For this review, take the finished solid that the model builds, in its own axes (mm). A direction names the side the tool comes from. Round coordinates to 2 decimals unless told otherwise and drop trailing zeros. Loops run counter-clockwise (first coordinate to the right, second up) from the corner with the lowest first, then second, coordinate; pieces in that order, holes last. Notation, with made-up numbers: M 69,71 L 106,71 A13 cw 106,79 Z; hole C -1,79.25 d1. An arc over 180 degrees is marked long. One line per question, with ' | ' between items. Start each with the question number.
1) For faces 5 (the face through (-1, -250, 42)), 6 (the face through (6, -30, -20)), 7 (the face through (-14, -140, 9)), list the 3-axis set-ups (+Z, -Z, +X, -X, +Y, -Y) from which the entire face can be reached by the end or side of a thin tool; tool diameter is ignored.
2) For pin 1 Ø5 at (x, y) = (-11.5, -99) entering from -Z; pin 2 Ø20 at (x, z) = (-17.5, 7.5) entering from -Y; pin 3 Ø2 at (x, y) = (-46.5, -216.5) entering from -Z, all flat-tipped, find the tip position at first contact; note any pin that passes through.
3) We need section C-C (y = -127). Give the boundary of the cut face in (x, z).
4) For probe 1 along Z at (x, y) = (2, -223.5); probe 2 along Z at (x, y) = (0, -29); probe 3 along Y at (x, z) = (34.5, -45.5), list the stretches that pass through material, from the lowest coordinate up. Write a range as from..to.
5) We need section A-A (x = 0). Give the boundary of the cut face in (y, z).
6) We need section B-B (z = 0). Give the boundary of the cut face in (x, y).
7) Mouldability with a two-part tool opening along Z and no side actions: class faces 1 (the face through (-1, -201, -30)), 2 (the face through (-4.336, -14.79, -19.524)), 3 (the face through (-14.985, -70.98, 0.66)), 4 (the face through (3, 0, 15)) as pulls with the +Z half, pulls with the -Z half, needs draft (parallel to the pull), parting line crosses it, or undercut.
8) We need section D-D (z = -23.5). Give the boundary of the cut face in (x, y).
```python
from build123d import *

# Parameters (mm, degrees)
F0_R     = 20
F1_DEPTH = 30
F2_R     = 30
F3_DEPTH = 40
F4_R     = 60
F5_DEPTH = 180
F6_R     = 15
F7_DEPTH = 250
F8_W     = 141.35922
F8_H     = 60
F9_DEPTH = 110
F10_R    = 10
F11_R    = 10


with BuildPart() as f1:
    # F0 (on Front) → F1 (new body)
    with BuildSketch(Plane.XZ):
        Circle(F0_R)
    extrude(amount=F1_DEPTH)

    # F2 (on face) → F3 (join)
    with BuildSketch(Plane.XZ.offset(30)):
        Circle(F2_R)
    extrude(amount=F3_DEPTH)

    # F4 (on face) → F5 (join)
    with BuildSketch(Plane.XZ.offset(70)):
        Circle(F4_R)
    extrude(amount=F5_DEPTH)

    # F6 (on face) → F7 (cut)
    with BuildSketch(Plane.XZ.offset(250)):
        Circle(F6_R)
    extrude(amount=-F7_DEPTH, mode=Mode.SUBTRACT)

    # F8 (on face) → F9 (cut)
    with BuildSketch(Plane.XZ.offset(250)):
        Rectangle(F8_W, F8_H)
    extrude(amount=-F9_DEPTH, mode=Mode.SUBTRACT)

    # F10
    f10_edges = [f1.edges().sort_by_distance(p)[0] for p in [
        (0, -140, 30),
    ]]
    fillet(f10_edges, radius=F10_R)

    # F11
    f11_edges = [f1.edges().sort_by_distance(p)[0] for p in [
        (0, -140, -30),
    ]]
    fillet(f11_edges, radius=F11_R)


solid = f1.part
```
Answers below:
1) face 5: +Z, -Z, +X, -X, -Y | face 6: +Y | face 7: +X, -X, -Y
2) pin 1: z = -59.32 | pin 2: y = -140 | pin 3: z = -39.11
3) outline: C 0,0 d120; hole C 0,0 d30
4) probe 1: -59.97..-30, 30..59.97 | probe 2: -20..-15, 15..20 | probe 3: -250..-70
5) outline: M -250,-60 L -70,-60 L -70,-30 L -30,-30 L -30,-20 L 0,-20 L 0,-15 L -140,-15 L -140,-20 A10 cw -150,-30 L -250,-30 Z; M -250,30 L -150,30 A10 cw -140,20 L -140,15 L 0,15 L 0,20 L -30,20 L -30,30 L -70,30 L -70,60 L -250,60 Z
6) outline: M -60,-140 L -15,-140 L -15,0 L -20,0 L -20,-30 L -30,-30 L -30,-70 L -60,-70 Z; M 15,-140 L 60,-140 L 60,-70 L 30,-70 L 30,-30 L 20,-30 L 20,0 L 15,0 Z
7) face 1: undercut | face 2: parting line crosses it | face 3: undercut | face 4: needs draft
8) outline: M -55.21,-140.63 L 55.21,-140.63 L 55.21,-70 L 18.65,-70 L 18.65,-30 L -18.65,-30 L -18.65,-70 L -55.21,-70 Z
